Design review of the part built by this model. Coordinates are the model's own, in mm. A direction names the side the tool comes from. Coordinates: 2 decimals unless noted, no trailing zeros. Loops run counter-clockwise (first coordinate to the right, second up) from the corner with the lowest first, then second, coordinate; pieces in that order, holes last. Notation, with made-up numbers: (67, 30.25) - (76, 30.25) arc R12 cw to (76, 50.25) - close; hole circle Ø11 at (46.25, 20.5). An arc over 180 degrees is marked (long way). Answer in a Markdown table with one row per item. Add a question column.
(1) We need section A-A, the plane z = 101. Write out the cut boundary in (x, y).
(2) The part is to be moulded in two halves that separate along X. For faces 4 (the face through (58.82, 94.48, 118.5)), 5 (the face through (1.963, 256.977, 59.16)), 6 (the face through (-86, -6.989, 59)), say which applies: released by +X, released by -X, zero draft, split by the parting line, or undercut.
(3) We need section B-B, the plane x = 85. Write out the cut boundary in (y, z), plus the area to 3 significant figures.
(4) To check wall thickness, follow L1, parallel to Y at x = 0, z = 89; L2, parallel to X at y = 5.5, z = 31; L3, parallel to X at y = 32, z = 50. State the ranges of each line that lie inside material, in increasing order. Write a range as [from, to].
(5) For faces 1 (the face through (-59.095, 96.44, 1.504)), 2 (the face through (-84, 7, 59)), 3 (the face through (71.54, 94.69, 59.16)), list the 3-axis set-ups (+Z, -Z, +X, -X, +Y, -Y) from which the entire face can be reached by the end or side of a thin tool; tool diameter is ignored.
(6) Clearance check with flat-ended pins moving along their axes: pin 1 (1 mm diameter, centred on x = -31, z = 79.5, fed in from +Y); pin 2 (4.5 mm diameter, centred on x = -85, z = 65.5, fed in from +Y); pin 3 (10 mm diameter, centred on x = 33.5, z = 85, fed in from -Y). State where each tip first meets the part, or that it passes through.
from build123d import *

# Parameters (mm, degrees)
PAD_DEPTH = 120
FILLET_R  = 5


with BuildPart() as part:
    # Sketch → Pad (new body)
    with BuildSketch(Plane.XY):
        with BuildLine():
            ThreePointArc((81.205589, 163.61348), (0, 257.000003), (-81.205589, 163.61348))
            Line((-61.604044, 23.818887), (-81.205589, 163.61348))
            ThreePointArc((-76.312668, 7), (-65.141068, 12.07111), (-61.604044, 23.818887))
            Line((-76.312668, 7), (-91.312668, 7))
            Line((-91.312668, 7), (-96.311409, -6.989133))
            Line((-76.311409, -6.989133), (-96.311409, -6.989133))
            ThreePointArc((-76.311409, -6.989133), (-54.584345, 2.892207), (-47.750327, 25.761451))
            Line((-67.341217, 165.557526), (-47.750327, 25.761451))
            ThreePointArc((67.341217, 165.557526), (0, 243.000004), (-67.341217, 165.557526))
            Line((67.341217, 165.557526), (47.739445, 25.762956))
            ThreePointArc((47.739445, 25.762956), (54.520356, 2.891123), (76.229044, -6.999999))
            Line((76.229044, -6.999999), (96.229044, -6.999999))
            Line((91.229042, 7.000001), (96.229044, -6.999999))
            Line((76.229042, 7.000001), (91.229042, 7.000001))
            ThreePointArc((61.603815, 23.818922), (65.084835, 12.077624), (76.229042, 7.000001))
            Line((81.205589, 163.61348), (61.603815, 23.818922))
        make_face()
    extrude(amount=PAD_DEPTH)

    # Fillet
    fillet_edges = [part.edges().sort_by_distance(p)[0] for p in [
        (54.520356, 2.891123, 0),
        (86.229044, -6.999999, 0),
        (86.229044, -6.999999, 120),
        (54.520356, 2.891123, 120),
        (57.540331, 95.660241, 0),
        (0, 243.000004, 0),
        (0, 243.000004, 120),
        (-57.545772, 95.659489, 0),
        (-54.584345, 2.892207, 0),
        (-86.311409, -6.989133, 0),
        (-86.311409, -6.989133, 120),
        (-54.584345, 2.892207, 120),
        (-57.545772, 95.659489, 120),
        (57.540331, 95.660241, 120),
    ]]
    fillet(fillet_edges, radius=FILLET_R)


solid = part.part
Responses:
| question | item | result |
|---|---|---|
| 1 | outline | (-96.31, -6.99) - (-76.31, -6.99) arc R28.83 ccw to (-47.75, 25.76) - (-67.34, 165.56) arc R68 cw (long way) to (67.34, 165.56) - (47.74, 25.76) arc R28.77 ccw to (76.23, -7) - (96.23, -7) - (91.23, 7) - (76.23, 7) arc R14.77 cw to (61.6, 23.82) - (81.21, 163.61) arc R82 ccw (long way) to (-81.21, 163.61) - (-61.6, 23.82) arc R14.84 cw to (-76.31, 7) - (-91.31, 7) - close |
| 2 | face 4 | undercut |
| 2 | face 5 | split by the parting line |
| 2 | face 6 | zero draft |
| 3 | outline | (-7, 5) arc R5 ccw to (-2, 0) - (7, 0) - (7, 120) - (-2, 120) arc R5 ccw to (-7, 115) - close |
| 3 | area | 1,670 mm2 |
| 4 | L1 | y = [243, 257] |
| 4 | L2 | x = [-91.85, -52.56], [52.5, 91.76] |
| 4 | L3 | x = [-62.75, -48.62], [48.61, 62.75] |
| 5 | face 1 | -Z |
| 5 | face 2 | +Z, -Z, -X |
| 5 | face 3 | +Z, -Z, +X |
| 6 | pin 1 | stops at y = 251.12 |
| 6 | pin 2 | stops at y = 7 |
| 6 | pin 3 | stops at y = 231.05 |
